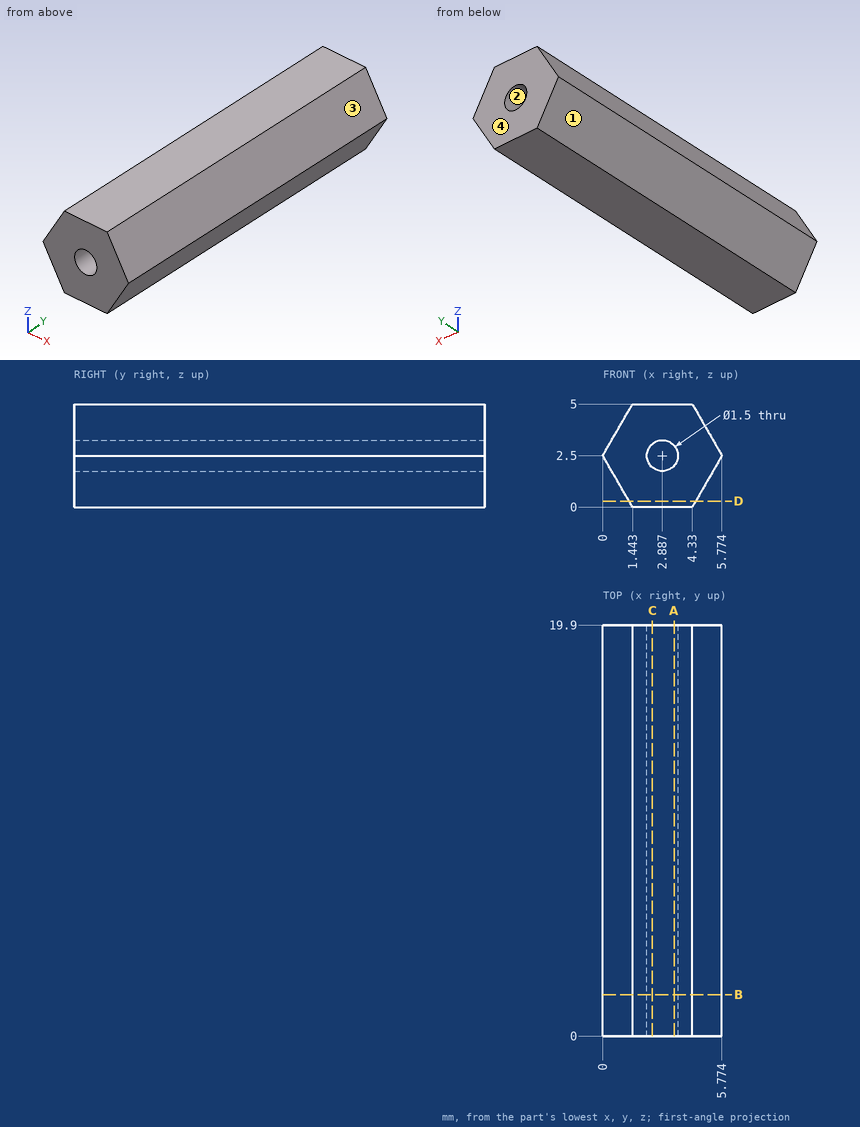
Can you work these out from the drawing? Everything is in mm from the part's minimum corner. Coordinates: 2 decimals unless noted, no trailing zeros. Loops run counter-clockwise (first coordinate to the right, second up) from the corner with the lowest first, then second, coordinate; pieces in that order, holes last. Notation, with made-up numbers: M 80,0.25 L 139,0.25 A28 ccw 139,26.25 Z; hole C 28,64 d8. An arc over 180 degrees is marked long. One line per item, written item: value.
1. Imagine slicing it at D-D (z = 0.3). List the corners of the cut face in (x, y) for me.
Geometry says:
outline: M 1.27,0 L 4.5,0 L 4.5,19.9 L 1.27,19.9 Z
2. Thinking about a two-plate mould opening in Z: for the marked faces 1, 2, 3 and 4, which applies, +Z half, -Z half, draft (parallel to the pull), parting line (faces both ways), or undercut?
Geometry says:
face 1: -Z half
face 2: undercut
face 3: +Z half
face 4: draft
3. Imagine slicing it at C-C (x = 2.4). List the corners of the cut face in (y, z) for me.
Geometry says:
outline: M 0,0 L 19.9,0 L 19.9,1.93 L 0,1.93 Z; M 0,3.07 L 19.9,3.07 L 19.9,5 L 0,5 Z
4. Will these pins go through, and if not, where does the flat tip stop? pin 1 Ø1 at (y, z) = (5, 4) entering from +X (1 decimal); pin 2 Ø1.5 at (y, z) = (13.5, 1.5) entering from +X; pin 3 Ø3 at (y, z) = (15.5, 1.5) entering from -X.
Geometry says:
pin 1: stops at x = 5.2
pin 2: stops at x = 5.63
pin 3: stops at x = 0
5. Imagine slicing it at B-B (y = 2). List the corners of the cut face in (x, z) for me.
Geometry says:
outline: M 0,2.5 L 1.44,0 L 4.33,0 L 5.77,2.5 L 4.33,5 L 1.44,5 Z; hole C 2.89,2.5 d1.5
6. Please list where these lines run through material, in increasing order: probe 1 along Z at (x, y) = (2.8, 10.5) (1 decimal); probe 2 along Z at (x, y) = (3.3, 4.5) (1 decimal); probe 3 along X at (y, z) = (2.5, 2.45) (1 decimal).
Geometry says:
probe 1: z = 0 to 1.8, 3.2 to 5
probe 2: z = 0 to 1.9, 3.1 to 5
probe 3: x = 0 to 2.1, 3.6 to 5.7
7. Imagine slicing it at A-A (x = 3.45). List the corners of the cut face in (y, z) for me (1 decimal).
Geometry says:
outline: M 0,0 L 19.9,0 L 19.9,2 L 0,2 Z; M 0,3 L 19.9,3 L 19.9,5 L 0,5 Z
